Verification items for the finished model (mm, model axes). Give positions to 0.01 mm unless a question says otherwise; leave off trailing zeros. Loops run counter-clockwise (first coordinate to the right, second up) from the corner with the lowest first, then second, coordinate; pieces in that order, holes last. Notation, with made-up numbers: (40, 88) -> (59, 88) arc R27 cw to (59, 118) -> close; hole circle Ø6 at (67, -4). An arc over 180 degrees is marked (long way). Answer in a Markdown table with one row per item. Add a question column.
Q1. Section check D-D on z = -25.5. Enter the section's corners in (x, y) (3 decimals).
Q2. Gauge pin test, flat ends, axial feed: P1, Ø0.8, axis at x = 22, y = 1.5, coming from the -Z side; P2, Ø1, axis at y = 1.5, z = 0, coming from the -X side; P3, Ø1.6, axis at y = 2, z = -0.5, coming from the +X side. Record the tip position at first contact, or that the pin passes through.
Q3. Section check C-C on y = 2.35. Enter the section's corners in (x, z) (1 decimal).
Q4. Section check A-A on z = 0. Enter the section's corners in (x, y) (3 decimals).
Q5. Section check B-B on x = 0. Enter the section's corners in (y, z) (3 decimals).
Q6. Material ranges on probe 1 along X at (y, z) = (0.6, 0.5) (3 decimals); probe 2 along X at (y, z) = (2.55, 1.5) (3 decimals); probe 3 along Z at (x, y) = (13, 3), recorded low to high.
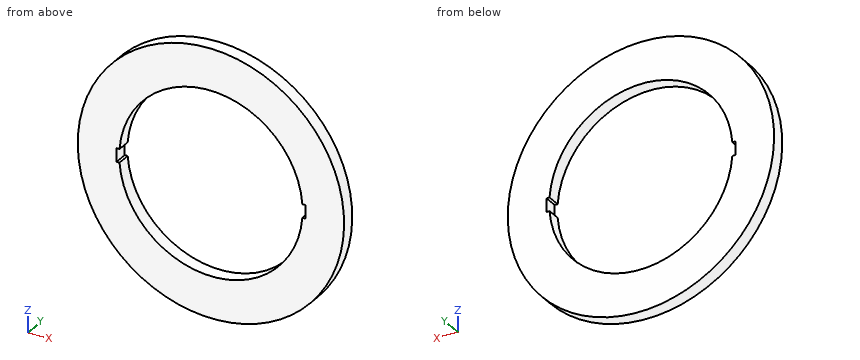
```python
from build123d import *

# Parameters (mm, degrees)
SKETCH1_R           = 31.369
BOSS_EXTRUDE1_DEPTH = 3.175


with BuildPart() as part:
    # Sketch1 → Boss-Extrude1 (new body)
    with BuildSketch(Plane(origin=(0, 0, 0), x_dir=(1, 0, 0), z_dir=(0, 1, 0))):
        with Locations(Location((0, 0, 0), (0, 0, 270))):
            Circle(SKETCH1_R)
        with BuildLine():
            Line((-22.225, 1.5875), (-21.531556928, 1.5875))
            ThreePointArc((-21.531556928, 1.5875), (0, 21.59), (21.531556928, 1.5875))
            Line((21.531556928, 1.5875), (22.225, 1.5875))
            Line((22.225, 1.5875), (22.225, -1.5875))
            Line((22.225, -1.5875), (21.531556928, -1.5875))
            ThreePointArc((21.531556928, -1.5875), (0, -21.59), (-21.531556928, -1.5875))
            Line((-21.531556928, -1.5875), (-22.225, -1.5875))
            Line((-22.225, -1.5875), (-22.225, 1.5875))
        make_face(mode=Mode.SUBTRACT)
    extrude(amount=BOSS_EXTRUDE1_DEPTH)


solid = part.part
```
Taken from the geometry:
| question | item | result |
|---|---|---|
| 1 | outline | (-18.269, 0) -> (18.269, 0) -> (18.269, 3.175) -> (-18.269, 3.175) -> close |
| 2 | P1 | stops at z = -22.75 |
| 2 | P2 | stops at x = -31.37 |
| 2 | P3 | stops at x = 31.37 |
| 3 | outline | circle Ø62.7 at (0, 0); hole (-22.2, -1.6) -> (-21.5, -1.6) arc R21.6 ccw to (21.5, -1.6) -> (22.2, -1.6) -> (22.2, 1.6) -> (21.5, 1.6) arc R21.6 ccw to (-21.5, 1.6) -> (-22.2, 1.6) -> close |
| 4 | outline | (-31.369, 0) -> (-22.225, 0) -> (-22.225, 3.175) -> (-31.369, 3.175) -> close; (22.225, 0) -> (31.369, 0) -> (31.369, 3.175) -> (22.225, 3.175) -> close |
| 5 | outline | (0, -31.369) -> (3.175, -31.369) -> (3.175, -21.59) -> (0, -21.59) -> close; (0, 21.59) -> (3.175, 21.59) -> (3.175, 31.369) -> (0, 31.369) -> close |
| 6 | probe 1 | x = -31.365 to -22.225, 22.225 to 31.365 |
| 6 | probe 2 | x = -31.333 to -22.225, 22.225 to 31.333 |
| 6 | probe 3 | z = -28.55 to -17.24, 17.24 to 28.55 |
